Could you check a few things on this drawing? It's one solid part, dimensions in mm from its lowest x, y, z. Coordinates: 2 decimals unless noted, no trailing zeros. Write each loop counter-clockwise with the first axis right and the second up, starting at its lowest first coordinate (ties: lowest second). Pieces come first, ordered by that corner, then holes. Notation, with made-up numbers: (48, -32) - (72, -32) arc R7 ccw to (72, -26) - close; hole circle Ø11 at (1, 65). An arc over 180 degrees is marked (long way). Answer as a JSON object with one key per item and string values. Group by question number.
1) Will this pin go through, and if not, where does the flat tip stop? pin 1 Ø5 at (x, y) = (8.5, 10.5) entering from -Z.
2) If we section it at A-A (y = 4): Write out the boundary of the cut face in (x, z).
3) If we section it at B-B (x = 4): Write out the boundary of the cut face in (y, z), plus the area to 3 significant figures.
4) Please list where these lines run through material, in increasing order: line 1 along Z through (x, y) = (4, 9.75); line 2 along X through (y, z) = (16.25, 10.75); line 3 along Z through (x, y) = (3.5, 12.75).
5) If we section it at C-C (z = 11.5): Write out the boundary of the cut face in (x, y), plus the area to 3 significant figures.
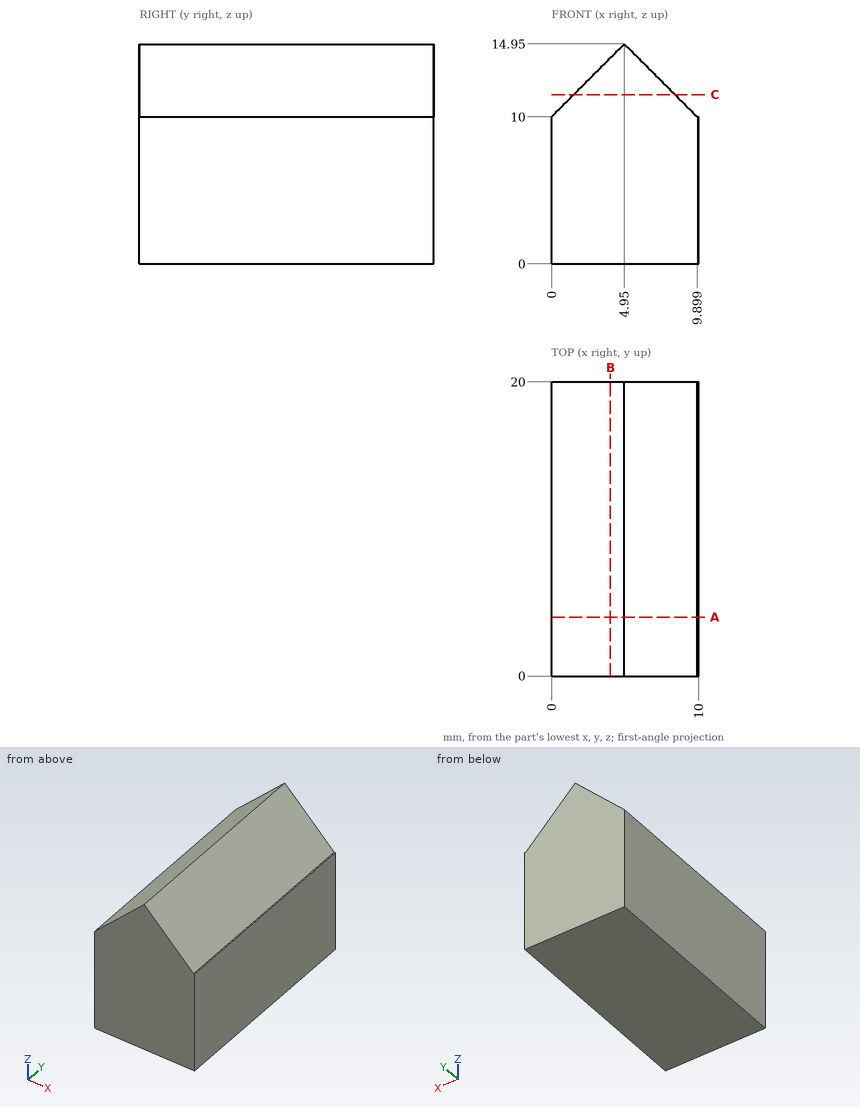
Here are the results:
{
 "1": {"pin 1": "stops at z = 0"},
 "2": {"outline": "(0, 0) - (10, 0) - (10, 10) - (9.9, 10) - (4.95, 14.95) - (0, 10) - close"},
 "3": {"outline": "(0, 0) - (20, 0) - (20, 14) - (0, 14) - close", "area": "280 mm²"},
 "4": {"line 1": "z = 0 to 14", "line 2": "x = 0.75 to 9.15", "line 3": "z = 0 to 13.5"},
 "5": {"outline": "(1.5, 0) - (8.4, 0) - (8.4, 20) - (1.5, 20) - close", "area": "138 mm²"}
}
